Geometry: final body of the model. Coordinates: model frame, mm. A direction names the side the tool comes from. Give positions to 0.01 mm unless a question says otherwise; leave off trailing zeros. Write each loop counter-clockwise with the first axis right and the second up, starting at its lowest first coordinate (ties: lowest second). Pieces come first, ordered by that corner, then holes. Notation, with made-up numbers: (67, 84) -> (85, 84) arc R20 cw to (85, 113) -> close; hole circle Ø1 at (73.25, 30.25). An arc over 180 degrees is marked (long way). Answer as a JSON object with one key per item and string values.
from build123d import *

# Parameters (mm, degrees)
F0_W     = 2600
F0_H     = 120
F1_DEPTH = 150
F3_DEPTH = 25
F5_DEPTH = 25
F7_R     = 25
F8_DEPTH = 3000


with BuildPart() as f1:
    # F0 (on Top) → F1 (new body)
    with BuildSketch(Plane.XY):
        with Locations((1300, 60)):
            Rectangle(F0_W, F0_H)
    extrude(amount=F1_DEPTH)

    # F2 (on Right) → F3 (join)
    with BuildSketch(Plane.YZ):
        with BuildLine():
            Line((26.7683122543, 230.984303782), (0, 150))
            Line((0, 150), (120, 150))
            Line((120, 150), (93.2316877457, 230.984303782))
            ThreePointArc((93.2316877457, 230.984303782), (60, 255), (26.7683122543, 230.984303782))
        make_face()
    extrude(amount=F3_DEPTH)


with BuildPart() as f5:
    # F4 (on face) → F5 (new body)
    with BuildSketch(Plane.YZ.offset(2600)):
        with BuildLine():
            Line((26.7683122543, 230.984303782), (0, 150))
            Line((0, 150), (120, 150))
            Line((120, 150), (93.2316877457, 230.984303782))
            ThreePointArc((93.2316877457, 230.984303782), (60, 255), (26.7683122543, 230.984303782))
        make_face()
    extrude(amount=-F5_DEPTH)


with BuildPart() as f1_1:
    add(f1.part)

    # F6: union F5
    add(f5.part)

    # F7 (on face) → F8 (cut)
    with BuildSketch(Plane.YZ.offset(2600)):
        with Locations((60, 220)):
            Circle(F7_R)
    extrude(amount=-F8_DEPTH, mode=Mode.SUBTRACT)


solid = f1_1.part
Q1. First-contact query: P1, Ø3, axis at x = 1784, y = 65.5, coming from the +Z side. Flat tip, straight axial feed; report the tip coordinate or a pass-through.
Values:
{"P1": "z = 150"}
Q2. Cut plane A-A (y = 60). Return the cut outline in (x, z), and give its area (3 significant figures).
Values:
{"outline": "(0, 0) -> (2600, 0) -> (2600, 195) -> (2575, 195) -> (2575, 150) -> (25, 150) -> (25, 195) -> (0, 195) -> close; (0, 245) -> (25, 245) -> (25, 255) -> (0, 255) -> close; (2575, 245) -> (2600, 245) -> (2600, 255) -> (2575, 255) -> close", "area": "393,000 mm²"}
Q3. Cut plane B-B (x = 543). Return the cut outline in (y, z), and give its area (3 significant figures).
Values:
{"outline": "(0, 0) -> (120, 0) -> (120, 150) -> (0, 150) -> close", "area": "18,000 mm²"}
Q4. Mould query, pull axis X, two halves, no side actions, for faces 1 (the flat face through (0, 59, 101)), 2 (the flat face through (25, 59, 192)), 3 (the flat face through (1282, 120, 74)). Classes: pulls with the +X half, pulls with the -X half, needs draft (parallel to the pull), parting line crosses it, or undercut.
Values:
{"face 1": "pulls with the -X half", "face 2": "undercut", "face 3": "needs draft"}
Q5. Material intervals for L1, parallel to X at y = 93.5, z = 216; L2, parallel to Z at x = 232.5, y = 36, sorted ascending. Write a range as from..to.
Values:
{"L1": "0..25, 2575..2600", "L2": "0..150"}
Q6. Set-up query: faces 4 (the cylindrical face through (12.675, 56.745, 244.787)), 5 (the flat face through (2575, 59, 192)). Return all of +Z, -Z, +X, -X, +Y, -Y with unobstructed straight access to the full face (end or side cutting, diameter ignored); none if empty.
Values:
{"face 4": "+X, -X", "face 5": "+Z, +Y, -Y"}
